from build123d import *

# Parameters (mm, degrees)
F2_R     = 8.471957502
F3_DEPTH = 5.6
F4_SIZE  = 1.09999
F5_SIZE  = 1
F6_SIZE  = 0.5
F7_R     = 0.5
F9_DEPTH = 1.6


# Not quite as in the source:
# - a fillet or chamfer is up to 0.001 mm smaller than in the source, because OpenCascade refuses the exact size


with BuildPart() as f1:
    # F0 (on Front) → F1 (revolve)
    with BuildSketch(Plane.XZ):
        Polygon((-58, 0), (0, 0), (0, 4), (-15, 4), (-15, 3.1), (-20, 3.1), (-20, 4.9), (-37.7, 4.9), (-37.7, 6), (-52.4, 6), (-52.4, 5), (-58, 5), align=None)
    revolve(axis=Axis((-31.3887451561, 0, 0), (-1, 0, 0)))

    # F2 (on face) → F3 (cut, through all)
    with BuildSketch(Plane(origin=(-58, 0, 0), x_dir=(0, -1, 0), z_dir=(-1, 0, 0))):
        Circle(F2_R)
        Polygon((-1.0790139268, 4.4909979157), (3.34981132, 3.1799524295), (4.4288252468, -1.3110454863), (1.0790139268, -4.4909979157), (-3.34981132, -3.1799524295), (-4.4288252468, 1.3110454863), align=None, mode=Mode.SUBTRACT)
    extrude(amount=-F3_DEPTH, mode=Mode.SUBTRACT)

    # F4 (size 1.1 in the source; OpenCascade refuses exactly that, so slightly less here)
    f4_edges = [f1.edges().sort_by_distance(p)[0] for p in [
        (-37.7, 0, -6),
    ]]
    chamfer(f4_edges, length=F4_SIZE)

    # F5
    f5_edges = [f1.edges().sort_by_distance(p)[0] for p in [
        (-52.4, 0, -6),
    ]]
    chamfer(f5_edges, length=F5_SIZE)

    # F6
    f6_edges = [f1.edges().sort_by_distance(p)[0] for p in [
        (0, 0, -4),
        (-15, 0, -4),
    ]]
    chamfer(f6_edges, length=F6_SIZE)

    # F7
    f7_edges = [f1.edges().sort_by_distance(p)[0] for p in [
        (-20, 0, -4.9),
    ]]
    fillet(f7_edges, radius=F7_R)

    # F8 (on face) → F9 (cut)
    with BuildSketch(Plane(origin=(-58, 0, 0), x_dir=(0, -1, 0), z_dir=(-1, 0, 0))):
        Polygon((-4.0528476409, -0.253822772), (-3.7257889258, -1.6150841712), (4.0528476409, 0.253822772), (3.7257889258, 1.6150841712), align=None)
    extrude(amount=-F9_DEPTH, mode=Mode.SUBTRACT)


solid = f1.part
For this review, take the finished solid that the model builds, in its own axes (mm). A direction names the side the tool comes from. Give positions to 0.01 mm unless a question says otherwise; leave off trailing zeros. Order: outer loops, then holes, each group sorted by start corner. A loop starts at its lowest first (then second) coordinate and runs counter-clockwise, first axis right, second up. Notation, with made-up numbers: (60, 63) -> (105, 63) arc R28 ccw to (105, 89) -> close; hole circle Ø11 at (77, -20.75). An arc over 180 degrees is marked (long way). Write item = value, one per line.
1) Draft analysis for pull direction Y (two halves, no side actions). For faces 1 (the face through (-29.22, -4.783, -1.062)), 2 (the face through (-55.24, 3.88, -0.97)), 3 (the face through (-52.4, 4.1, -0.8)), 4 (the face through (-57.211, 0.109, 0.694)), state which applies: pulls with the +Y half, pulls with the -Y half, needs draft (parallel to the pull), parting line crosses it, or undercut.
Findings:
face_1 = parting line crosses it
face_2 = pulls with the +Y half
face_3 = needs draft
face_4 = undercut
2) To check wall thickness, follow L1, parallel to X at y = 1.75, z = -0.5; L2, parallel to X at y = 3.5, z = -2; L3, parallel to Z at x = -2, y = 0.25. State the ranges of each line that lie inside material, in increasing order. Write a range as from..to.
Findings:
L1 = -56.4..0
L2 = -58..-20
L3 = -3.99..3.99
3) For faces 5 (the face through (-20, -3, -2)), 6 (the face through (-55.239, 1.104, -3.845)), 7 (the face through (-55.239, 2.777, 2.879)), 8 (the face through (-55.239, -1.104, 3.845)), list the 3-axis set-ups (+Z, -Z, +X, -X, +Y, -Y) from which the entire face can be reached by the end or side of a thin tool; tool diameter is ignored.
Findings:
face_5 = none
face_6 = -Z, -X, +Y
face_7 = +Z, -X, +Y
face_8 = +Z, -X, -Y
4) We need section C-C, the plane x = -34.5. Give the boundary of the cut face in (y, z).
Findings:
outline = circle Ø9.8 at (0, 0)
5) Insertion check: pin 1 (4 mm diameter, centred on x = -7.5, y = -3, fed in from -Z); pin 2 (5 mm diameter, centred on x = -17, y = -3.5, fed in from -Z); pin 3 (2 mm diameter, centred on y = 3, z = -4.5, fed in from -X). Each pin has a flat end and moves straight along its axis. Give the tip position at first contact, or say it passes through.
Findings:
pin_1 = -3.87
pin_2 = -2.93
pin_3 = -52.4
6) We need section B-B, the plane x = -19.5. Give the boundary of the cut face in (y, z), and give its area (3 significant figures).
Findings:
outline = circle Ø6.2 at (0, 0)
area = 30.2 mm^2
